Read the model definition and answer for the solid it produces. Units are mm, in the model's axes. Give positions to 0.01 mm unless a question says otherwise; leave off trailing zeros. Write each loop counter-clockwise with the first axis right and the second up, starting at its lowest first coordinate (ties: lowest second). Pieces come first, ordered by that corner, then holes. Notation, with made-up numbers: (6.5, -10.75) -> (38.5, -10.75) arc R11 cw to (38.5, 1.25) -> close; hole circle Ø9 at (-8.75, 30). An arc over 180 degrees is marked (long way). Write item = value, one per line.
Autodesk Inventor part; units mm, degrees
ref_plane "YZ Plane" through (0, 0, 0) normal (1, 0, 0) x (0, 1, 0)
ref_plane "XZ Plane" through (0, 0, 0) normal (0, 1, 0) x (-1, 0, 0)
ref_plane "XY Plane" through (0, 0, 0) normal (0, 0, 1) x (1, 0, 0)
sketch "Sketch1" plane through (0, 0, 0) normal (0, 0, 1) x (1, 0, 0)
  line L0 (456.5044, 429.8855) -> (462.0044, 429.8855)
  line L1 (462.0044, 429.8855) -> (462.0044, 389.8855)
  line L2 (462.0044, 389.8855) -> (456.5044, 389.8855)
  line L3 (456.5044, 389.8855) -> (456.5044, 339.8855)
  line L4 (456.5044, 339.8855) -> (462.0044, 339.8855)
  line L5 (462.0044, 339.8855) -> (462.0044, 339.8855)
  line L6 (22.5044, 429.8855) -> (17.0044, 429.8855)
  line L7 (17.0044, 429.8855) -> (17.0044, 389.8855)
  line L8 (17.0044, 389.8855) -> (22.5044, 389.8855)
  line L9 (22.5044, 389.8855) -> (22.5044, 339.8855)
  line L10 (22.5044, 339.8855) -> (17.0044, 339.8855)
  line L11 (17.0044, 339.8855) -> (17.0044, 339.8855)
  line L12 (17.0044, 339.8855) -> (462.0044, 339.8855)
  line L13 (22.5044, 559.8855) -> (159.5044, 559.8855)
  line L14 (159.5044, 559.8855) -> (159.5044, 565.3855)
  line L15 (456.5044, 559.8855) -> (319.5044, 559.8855)
  line L16 (319.5044, 559.8855) -> (319.5044, 565.3855)
  line L17 (319.5044, 565.3855) -> (159.5044, 565.3855)
  circle A0 centre (174.5044, 552.1705) radius 2
  circle A1 centre (304.5044, 552.1705) radius 2
  line L18 (22.5044, 429.8855) -> (22.5044, 479.8855)
  line L19 (22.5044, 479.8855) -> (17.0044, 479.8855)
  line L20 (17.0044, 479.8855) -> (17.0044, 519.8855)
  line L21 (17.0044, 519.8855) -> (22.5044, 519.8855)
  line L22 (22.5044, 559.8855) -> (22.5044, 519.8855)
  line L23 (22.5044, 479.8855) -> (22.5044, 429.8855)
  line L24 (456.5044, 479.8855) -> (462.0044, 479.8855)
  line L25 (462.0044, 479.8855) -> (462.0044, 519.8855)
  line L26 (462.0044, 519.8855) -> (456.5044, 519.8855)
  line L27 (456.5044, 559.8855) -> (456.5044, 519.8855)
  line L28 (456.5044, 479.8855) -> (456.5044, 429.8855)
  circle A2 centre (105.5044, 349.8855) radius 2
  circle A3 centre (151.0044, 349.8855) radius 2
  circle A4 centre (128.2544, 349.8855) radius 2
  circle A5 centre (328.0044, 349.8855) radius 2
  circle A6 centre (350.7544, 349.8855) radius 2
  circle A7 centre (373.5044, 349.8855) radius 2
  circle A8 centre (31.0044, 504.8855) radius 2
  circle A9 centre (31.0044, 354.8855) radius 2
  circle A10 centre (448.0044, 504.8855) radius 2
  circle A11 centre (448.0044, 354.8855) radius 2
  dimension "d105" = 50
  dimension "d148" = 445
  dimension "d196" = 137
  dimension "d197" = 137
  dimension "d199" = 4
  dimension "d200" = 4
  dimension "d203" = 7.715
  dimension "d204" = 7.715
  dimension "d207" = 5.5
  dimension "d209" = 5.5
  dimension "d211" = 5.5
  dimension "d214" = 4
  dimension "d215" = 4
  dimension "d216" = 4
  dimension "d217" = 4
  dimension "d218" = 4
  dimension "d219" = 4
  dimension "d221" = 22.75
  dimension "d222" = 22.75
  dimension "d224" = 22.75
  dimension "d225" = 22.75
  dimension "d226" = 4
  dimension "d227" = 4
  dimension "d234" = 90
  dimension "d235" = 90
  dimension "d236" = 90
  dimension "d238" = 55
  dimension "d244" = 160
  dimension "d245" = 5.5
  dimension "d246" = 5.5
  dimension "d247" = 5.5
  dimension "d248" = 5.5
  dimension "d249" = 5.5
  dimension "d250" = 5.5
  dimension "d251" = 8.5
  dimension "d252" = 8.5
  dimension "d253" = 150
  dimension "d254" = 152
  dimension "d255" = 152
  dimension "d256" = 55
  dimension "d257" = 8.5
  dimension "d258" = 4
  dimension "d259" = 8.5
  dimension "d260" = 150
  dimension "d261" = 10
  dimension "d262" = 10
  dimension "d263" = 10
  dimension "d264" = 10
  dimension "d265" = 10
  dimension "d266" = 10
  dimension "d269" = 40
  dimension "d270" = 40
  dimension "d271" = 40
  dimension "d272" = 50
  dimension "d273" = 40
  dimension "d274" = 40
  dimension "d275" = 50
  dimension "d276" = 40
  dimension "d277" = 50
  dimension "d280" = 0
  dimension "d281" = 0
  dimension "d282" = 0
  dimension "d283" = 90
  dimension "d284" = 90
extrude "Extrusion1" add sketch "Sketch1" along normal blind 5.5
properties part number "Techo Carcasa" material "MDF Medium Density Fiberboard"
(1) Consider L1, parallel to Y at x = 390.5, z = 3.9; L2, parallel to X at y = 527.5, z = 1; L3, parallel to Y at x = 107, z = 1.65. Determine where each line is inside the solid, lowest interval first.
Checks:
L1 = 339.89 to 559.89
L2 = 22.5 to 456.5
L3 = 339.89 to 348.56, 351.21 to 559.89
(2) Given P1, Ø3, axis at x = 407.5, z = 2.5, coming from the +Y side; P2, Ø3, axis at x = 20.5, z = 3.5, coming from the -Y side; P3, Ø3, axis at x = 458.5, z = 2, coming from the +Y side, each flat-ended and moving along its own axis, determine where each tip first touches the part or whether it passes through.
Checks:
P1 = 559.89
P2 = 389.89
P3 = 519.89
(3) The part is cut by section B-B on z = 3.8. Count the separate pieces of the cut face and the enclosed holes in it, plus the area to 3 significant figures.
Checks:
separate_pieces = 1
enclosed_holes = 12
area = 97,100 mm²
(4) The part is cut by section A-A on x = 379.5. Determine the outline of the cut face in (y, z), plus the area to 3 significant figures.
Checks:
outline = (339.89, 0) -> (559.89, 0) -> (559.89, 5.5) -> (339.89, 5.5) -> close
area = 1,210 mm²
(5) The part is cut by section C-C on y = 457.5. Determine the outline of the cut face in (x, z), plus the area to 3 significant figures.
Checks:
outline = (22.5, 0) -> (456.5, 0) -> (456.5, 5.5) -> (22.5, 5.5) -> close
area = 2,390 mm²
